Build history of the part. All positions in model axes, mm. A direction names the side the tool comes from. Coordinates: 2 decimals unless noted, no trailing zeros. Write each loop counter-clockwise with the first axis right and the second up, starting at its lowest first coordinate (ties: lowest second). Pieces come first, ordered by that corner, then holes.
```python
from build123d import *

# Parameters (mm, degrees)
SKETCH2_W                          = 45
SKETCH2_H                          = 40
STEPPER_SLIDER_BOSS_EXTRUDE1_DEPTH = 8
SKETCH1_R                          = 1.75
STEPPER_HOLE_CUT_EXTRUDE1_DEPTH    = 8


with BuildPart() as part:
    # Sketch2 → Stepper Slider Boss-Extrude1 (new body)
    with BuildSketch(Plane(origin=(0, 0, 0), x_dir=(1, 0, 0), z_dir=(0, 1, 0))):
        with Locations((-2.5, -2.5)):
            Rectangle(SKETCH2_W, SKETCH2_H)
    extrude(amount=-STEPPER_SLIDER_BOSS_EXTRUDE1_DEPTH)

    # Sketch1 → Stepper Hole Cut-Extrude1 (cut)
    with BuildSketch(Plane(origin=(0, 0, 0), x_dir=(1, 0, 0), z_dir=(0, 1, 0))):
        with Locations(Location((-18.45, -1.75, 0), (0, 0, 270))):
            Circle(SKETCH1_R)
        with Locations(Location((16.95, -7.041502622, 0), (0, 0, 270))):
            Circle(SKETCH1_R)
        with Locations(Location((-16.95, -7.041502622, 0), (0, 0, 270))):
            Circle(SKETCH1_R)
        with BuildLine():
            Line((8.75, -17.928746497), (8.75, -10.928746497))
            ThreePointArc((8.75, -10.928746497), (0, 14), (-8.75, -10.928746497))
            Line((-8.75, -10.928746497), (-8.75, -17.928746497))
            Line((-8.75, -17.928746497), (8.75, -17.928746497))
        make_face()
    extrude(amount=-STEPPER_HOLE_CUT_EXTRUDE1_DEPTH, mode=Mode.SUBTRACT)


solid = part.part
```
1. 3-axis set-ups, long thin cutter, end or side, ignore diameter. For faces 1 (the face through (-13, -8, 7)), 2 (the face through (0, -4, 17.929)): which of +Z, -Z, +X, -X, +Y, -Y reach the whole face in a straight line?
Computed values:
face 1: +Z, -Z, +X, -X, -Y
face 2: +Y, -Y
2. Saw through at D-D on z = 1.75. List the corners of the cut face in (x, y), plus the area to 3 significant figures.
Computed values:
outline: (-25, -8) - (-20.2, -8) - (-20.2, 0) - (-25, 0) - close; (-16.7, -8) - (-13.89, -8) - (-13.89, 0) - (-16.7, 0) - close; (13.89, -8) - (20, -8) - (20, 0) - (13.89, 0) - close
area: 110 mm2
3. Flat gauge pin, fed straight in: pin 1 (17 mm diameter, centred on x = 0, z = 0, fed in from +Y). Where does the tip first touch, or does it go through?
Computed values:
pin 1: passes through
4. Saw through at C-C on z = 16. List the corners of the cut face in (x, y).
Computed values:
outline: (-25, -8) - (-8.75, -8) - (-8.75, 0) - (-25, 0) - close; (8.75, -8) - (20, -8) - (20, 0) - (8.75, 0) - close
5. Saw through at A-A on x = 0. List the corners of the cut face in (y, z), plus the area to 3 significant figures.
Computed values:
outline: (-8, -17.5) - (0, -17.5) - (0, -14) - (-8, -14) - close; (-8, 17.93) - (0, 17.93) - (0, 22.5) - (-8, 22.5) - close
area: 64.6 mm2
6. Saw through at B-B on y = -2.5. List the corners of the cut face in (x, z), plus the area to 3 significant figures.
Computed values:
outline: (-25, -17.5) - (20, -17.5) - (20, 22.5) - (-25, 22.5) - close; hole circle Ø3.5 at (-18.45, 1.75); hole circle Ø3.5 at (-16.95, 7.04); hole (-8.75, 10.93) arc R14 ccw (long way) to (8.75, 10.93) - (8.75, 17.93) - (-8.75, 17.93) - close; hole circle Ø3.5 at (16.95, 7.04)
area: 1,070 mm2
7. Probe line 1 along X through (y, z) = (-1, 17); line 2 along X through (y, z) = (-7, 1); line 3 along X through (y, z) = (-2.75, -7). List the from-to ranges inside material, lowest first.
Computed values:
line 1: x = -25 to -8.75, 8.75 to 20
line 2: x = -25 to -20.03, -16.87 to -13.96, 13.96 to 20
line 3: x = -25 to -12.12, 12.12 to 20
8. Mould opens along Z. For faces 3 (the face through (-8.75, -4, 14)), 4 (the face through (-3, -4, -17.5)), 5 (the face through (-3, -4, 22.5)) say: +Z half, -Z half, draft (parallel to the pull), parting line (faces both ways), or undercut.
Computed values:
face 3: undercut
face 4: -Z half
face 5: +Z half
